Could you check a few things on this model? Use its own coordinates, in mm. A direction names the side the tool comes from. Give positions to 0.01 mm unless a question says otherwise; leave off trailing zeros. Order: outer loops, then holes, each group sorted by start corner. A loop starts at its lowest first (then second) coordinate and runs counter-clockwise, first axis right, second up. Notation, with made-up numbers: (43.25, -4) -> (47.25, -4) arc R18 cw to (47.25, 15) -> close; hole circle Ø1 at (67, 68). An arc over 180 degrees is marked (long way). One line per item, written item: value.
```python
from build123d import *

# Parameters (mm, degrees)
F0_W        = 80
F0_H        = 26
F0_R        = 6
F0_R_2      = 4
F1_DEPTH    = 13
F2_T        = 2.5
F2_T3_DEPTH = 31
F3_R        = 9.5
F3_R_2      = 4
F4_DEPTH    = 50
F5_R        = 2.49999


# Not quite as in the source:
# - a fillet or chamfer is up to 0.001 mm smaller than in the source, because OpenCascade refuses the exact size
# - a shell that OpenCascade refuses in one call is made with other operations: the cavity is built on its own and cut out


with BuildPart() as f1:
    # F0 (on Front) → F1 (new body, symmetric)
    with BuildSketch(Plane.XZ):
        Polygon((0, 25.9917649148), (0, 59.9917649148), (-26, 59.9917649148), (-26, -40.0082350852), (0, -40.0082350852), (0, -0.0082350852), align=None)
        with Locations((40, 12.9917649148)):
            Rectangle(F0_W, F0_H)
        with Locations((10, 7.9917649148)):
            Circle(F0_R, mode=Mode.SUBTRACT)
        with Locations((68, 12.9917649148)):
            Circle(F0_R_2, mode=Mode.SUBTRACT)
    extrude(amount=F1_DEPTH, both=True)

    # F2: shell of thickness 2.5, made by hand


with BuildPart() as f2_core1:
    # F2_t2: copy of F1
    add(f1.part)

    # the walls: a layer under each face that stays
    f2_faces = [f2_core1.faces().sort_by_distance(p)[0] for p in [
        (0, 0, 42.9917649148),
        (40, 0, 25.9917649148),
        (80, 0, 12.9917649148),
        (40, 0, -0.0082350852),
        (0, 0, -20.0082350852),
        (-26, 0, 9.9917649148),
        (27, -13, 9.9917649148),
        (4, 0, 7.9917649148),
        (64, 0, 12.9917649148),
        (27, 13, 9.9917649148),
    ]]
    thicken(f2_faces, amount=-F2_T, mode=Mode.SUBTRACT)

    # F2_s4 → F2_t3 (cut)
    with BuildSketch(Plane.XZ.offset(-15.5)):
        Polygon((0.025, 26.0167649148), (-2.5, 25.9917649148), (-2.5, 23.4917649148), (0, 23.4917649148), align=None)
        Polygon((0.025, -0.0332350852), (0, 2.4917649148), (-2.5, 2.4917649148), (-2.5, -0.0082350852), align=None)
    extrude(amount=F2_T3_DEPTH, mode=Mode.SUBTRACT)


with BuildPart() as f1_1:
    add(f1.part)

    # what is left inside the walls is the cavity
    f2_cavity = [f2_core1.part.solids().sort_by_distance(p)[0] for p in [
        (-10.875, 10.475, 4.436209),
    ]]
    add(f2_cavity, mode=Mode.SUBTRACT)

    # F3 (on Top) → F4 (cut, symmetric)
    with BuildSketch(Plane.XY):
        with Locations((55, 0)):
            Circle(F3_R)
        with Locations((38.5, 0)):
            Circle(F3_R_2)
    extrude(amount=F4_DEPTH, both=True, mode=Mode.SUBTRACT)

    # F5 (radius 2.5 in the source; OpenCascade refuses exactly that, so slightly less here)
    f5_edges = [f1_1.edges().sort_by_distance(p)[0] for p in [
        (0, 0, 59.991765),
        (-13, -13, 59.991765),
        (-13, 13, 59.991765),
        (-26, 0, 59.991765),
        (-26, 0, -40.008235),
        (-13, 13, -40.008235),
        (0, 0, -40.008235),
        (-13, -13, -40.008235),
    ]]
    fillet(f5_edges, radius=F5_R)


solid = f1_1.part
```
1) If I drill on line 1 along Y through (x, z) = (54, 4.5); line 2 along Z through (x, y) = (10, -4.25); line 3 along Y through (x, z) = (38.5, 25.1), over which ranges is the centre line in solid material (lowest first)?
Answer below:
line 1: y = -13 to -10.5, 10.5 to 13
line 2: z = -0.01 to 1.99, 13.99 to 16.49, 23.49 to 25.99
line 3: y = -13 to -4, 4 to 13
2) Suppose I cut it at D-D, the plane z = -20. Write out the boundary of the cut face in (x, y), then the cut area to 3 significant figures.
Answer below:
outline: (-26, -13) -> (0, -13) -> (0, 13) -> (-26, 13) -> close; hole (-23.5, -10.5) -> (-2.5, -10.5) -> (-2.5, 10.5) -> (-23.5, 10.5) -> close
area: 235 mm2
3) Suppose I cut it at A-A, the plane x = 68. Write out the boundary of the cut face in (y, z), then the cut area to 3 significant figures.
Answer below:
outline: (-13, -0.01) -> (13, -0.01) -> (13, 8.99) -> (-13, 8.99) -> close; (-13, 16.99) -> (13, 16.99) -> (13, 25.99) -> (-13, 25.99) -> close; hole (-10.5, 2.49) -> (10.5, 2.49) -> (10.5, 6.49) -> (-10.5, 6.49) -> close; hole (-10.5, 19.49) -> (10.5, 19.49) -> (10.5, 23.49) -> (-10.5, 23.49) -> close
area: 300 mm2
4) We'd pull the mould along Y, two halves only. Please class faces 1 (the cylindrical face through (-0.752, 0.182, 59.279)), 2 (the cylindrical face through (-13.182, 12.248, 59.279)), 3 (the flat face through (28, 0, 23.492)), 4 (the flat face through (46.6, -4.8, 2.492)): +Y half, -Y half, draft (parallel to the pull), parting line (faces both ways), or undercut.
Answer below:
face 1: draft
face 2: +Y half
face 3: undercut
face 4: undercut
5) Suppose I cut it at B-B, the plane x = 10. Write out the boundary of the cut face in (y, z), then the cut area to 3 significant figures.
Answer below:
outline: (-13, -0.01) -> (13, -0.01) -> (13, 1.99) -> (-13, 1.99) -> close; (-13, 13.99) -> (13, 13.99) -> (13, 25.99) -> (-13, 25.99) -> close; hole (-10.5, 16.49) -> (10.5, 16.49) -> (10.5, 23.49) -> (-10.5, 23.49) -> close
area: 217 mm2
6) For P1, Ø5, axis at y = -6.5, z = 49.5, coming from the +X side; P2, Ø13, axis at x = 47.5, y = -2, coming from the -Z side; P3, Ø10, axis at x = 46, y = 1, coming from the +Z side, each with a flat end and sliding along its axis, tell me the tip position at first contact or that it passes through.
Answer below:
P1: stops at x = 0
P2: stops at z = -0.01
P3: stops at z = 25.99
7) Suppose I cut it at C-C, the plane x = 38.5. Write out the boundary of the cut face in (y, z).
Answer below:
outline: (-13, -0.01) -> (-4, -0.01) -> (-4, 2.49) -> (-10.5, 2.49) -> (-10.5, 23.49) -> (-4, 23.49) -> (-4, 25.99) -> (-13, 25.99) -> close; (4, -0.01) -> (13, -0.01) -> (13, 25.99) -> (4, 25.99) -> (4, 23.49) -> (10.5, 23.49) -> (10.5, 2.49) -> (4, 2.49) -> close
8) For faces 5 (the flat face through (8, 10.5, 18)), 6 (the flat face through (-2.5, 0, -18)), 7 (the flat face through (14, 13, 21)), 8 (the flat face through (39, -6, -0.008)), which set-ups out of +Z, -Z, +X, -X, +Y, -Y let a thin tool reach every point of the face, with its end or its side?
Answer below:
face 5: none
face 6: +Z, -Z
face 7: +Z, -Z, +X, -X, +Y
face 8: -Z, +X, +Y, -Y
